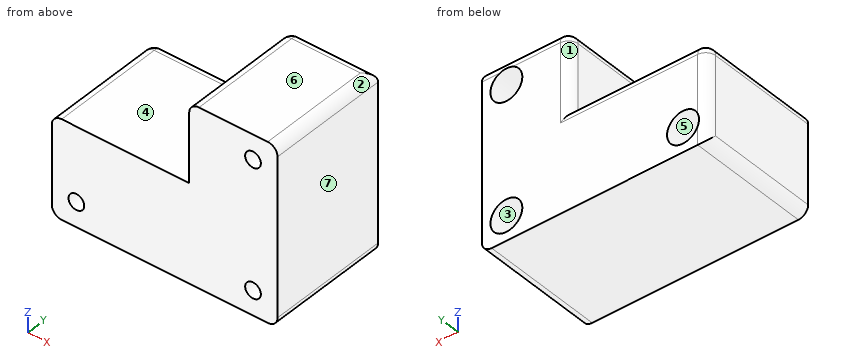
from build123d import *

# Parameters (mm, degrees)
F0_R         = 3.25
F0_R_2       = 1.6
F0_W         = 26
F0_H         = 2
F1_DEPTH     = 25
F2_DEPTH     = 15
F3_T1_DEPTH  = 23
F3_T3_DEPTH  = 21
F3_T5_DEPTH  = 28
F3_T7_DEPTH  = 35
F3_T9_DEPTH  = 26
F3_T11_DEPTH = 14
F3_S15_W     = 2
F3_S15_H     = 2
F3_T16_DEPTH = 2
F3_S21_W     = 2
F3_S21_H     = 2
F3_T22_DEPTH = 2
F3_T29_DEPTH = 31
F3_T33_DEPTH = 19


# Not quite as in the source:
# - a fillet or chamfer that OpenCascade refuses, or shapes differently, is made with other operations: its cross-section is extruded or revolved along the edge and cut away or added


with BuildPart() as f1:
    # F0 (on Front) → F1 (new body)
    with BuildSketch(Plane.XZ):
        Polygon((-23, 0), (-23, -18), (23, -18), (23, 18), (5, 18), (5, 2), (3, 2), (3, 0), align=None)
        with Locations((-18, -13)):
            Circle(F0_R, mode=Mode.SUBTRACT)
        with Locations((18, -13)):
            Circle(F0_R, mode=Mode.SUBTRACT)
        with Locations((18, 13)):
            Circle(F0_R, mode=Mode.SUBTRACT)
        with Locations((18, 13)):
            Circle(F0_R)
        with Locations((18, 13)):
            Circle(F0_R_2, mode=Mode.SUBTRACT)
        with Locations((18, -13)):
            Circle(F0_R)
        with Locations((18, -13)):
            Circle(F0_R_2, mode=Mode.SUBTRACT)
        with Locations((-18, -13)):
            Circle(F0_R)
        with Locations((-18, -13)):
            Circle(F0_R_2, mode=Mode.SUBTRACT)
        with Locations((-10, 1)):
            Rectangle(F0_W, F0_H)
    extrude(amount=F1_DEPTH)

    # F0 (on Front) → F2 (cut)
    with BuildSketch(Plane.XZ):
        with Locations((18, -13)):
            Circle(F0_R)
        with Locations((18, -13)):
            Circle(F0_R_2, mode=Mode.SUBTRACT)
        with Locations((-18, -13)):
            Circle(F0_R)
        with Locations((-18, -13)):
            Circle(F0_R_2, mode=Mode.SUBTRACT)
        with Locations((18, 13)):
            Circle(F0_R)
        with Locations((18, 13)):
            Circle(F0_R_2, mode=Mode.SUBTRACT)
    extrude(amount=F2_DEPTH, mode=Mode.SUBTRACT)

    # F3: fillet of radius 2 on 9 edges, made by hand

    # F3_s2 → F3_t1 (cut)
    with BuildSketch(Plane.XY.offset(-23)):
        with BuildLine():
            ThreePointArc((-23, -2), (-22.4142135624, -0.5857864376), (-21, 0))
            Line((-21, 0), (-23, 0))
            Line((-23, 0), (-23, -2))
        make_face()
    extrude(amount=F3_T1_DEPTH, mode=Mode.SUBTRACT)

    # F3_s4 → F3_t3 (cut)
    with BuildSketch(Plane.YZ.offset(7)):
        with BuildLine():
            ThreePointArc((0, 16), (-0.5857864376, 17.4142135624), (-2, 18))
            Line((-2, 18), (0, 18))
            Line((0, 18), (0, 16))
        make_face()
    extrude(amount=F3_T3_DEPTH, mode=Mode.SUBTRACT)

    # F3_s6 → F3_t5 (cut)
    with BuildSketch(Plane.XZ.offset(2)):
        with BuildLine():
            ThreePointArc((-23, 0), (-22.4142135624, 1.4142135624), (-21, 2))
            Line((-21, 2), (-23, 2))
            Line((-23, 2), (-23, 0))
        make_face()
        with BuildLine():
            ThreePointArc((7, 18), (5.5857864376, 17.4142135624), (5, 16))
            Line((5, 16), (5, 18))
            Line((5, 18), (7, 18))
        make_face()
    extrude(amount=F3_T5_DEPTH, mode=Mode.SUBTRACT)

    # F3_s8 → F3_t7 (cut)
    with BuildSketch(Plane.XZ.offset(-5)):
        with BuildLine():
            ThreePointArc((-21, -18), (-22.4142135624, -17.4142135624), (-23, -16))
            Line((-23, -16), (-23, -18))
            Line((-23, -18), (-21, -18))
        make_face()
        with BuildLine():
            ThreePointArc((21, -18), (22.4142135624, -17.4142135624), (23, -16))
            Line((23, -16), (23, -18))
            Line((23, -18), (21, -18))
        make_face()
        with BuildLine():
            ThreePointArc((23, 16), (22.4142135624, 17.4142135624), (21, 18))
            Line((21, 18), (23, 18))
            Line((23, 18), (23, 16))
        make_face()
    extrude(amount=F3_T7_DEPTH, mode=Mode.SUBTRACT)

    # F3_s10 → F3_t9 (cut)
    with BuildSketch(Plane.YZ.offset(-21)):
        with BuildLine():
            ThreePointArc((0, 0), (-0.5857864376, 1.4142135624), (-2, 2))
            Line((-2, 2), (0, 2))
            Line((0, 2), (0, 0))
        make_face()
    extrude(amount=F3_T9_DEPTH, mode=Mode.SUBTRACT)

    # F3_s12 → F3_t11 (cut)
    with BuildSketch(Plane.XY.offset(2)):
        with BuildLine():
            ThreePointArc((7, 0), (5.5857864376, -0.5857864376), (5, -2))
            Line((5, -2), (5, 0))
            Line((5, 0), (7, 0))
        make_face()
    extrude(amount=F3_T11_DEPTH, mode=Mode.SUBTRACT)


with BuildPart() as f3_tool14:
    # F3_s15 → F3_t16 (new body)
    with BuildSketch(Plane.YZ.offset(-21)):
        with Locations((-1, 1)):
            Rectangle(F3_S15_W, F3_S15_H)
    extrude(amount=-F3_T16_DEPTH)

    # F3_s17 → F3_t18 (revolve, cut)
    with BuildSketch(Plane(origin=(-21, -2, 0), x_dir=(0, -0.7071067812, -0.7071067812), z_dir=(0, 0.7071067812, -0.7071067812))):
        with BuildLine():
            ThreePointArc((0, -2), (2, 0), (0, 2))
            Line((0, 2), (0, -2))
        make_face()
    revolve(axis=Axis((-21, -2, 0), (-1, 0, 0)), mode=Mode.SUBTRACT)


with BuildPart() as f1_1:
    add(f1.part)

    # F3_t13: cut F3_tool14
    add(f3_tool14.part, mode=Mode.SUBTRACT)


with BuildPart() as f3_tool20:
    # F3_s21 → F3_t22 (new body)
    with BuildSketch(Plane.XZ.offset(2)):
        with Locations((6, 17)):
            Rectangle(F3_S21_W, F3_S21_H)
    extrude(amount=-F3_T22_DEPTH)

    # F3_s23 → F3_t24 (revolve, cut)
    with BuildSketch(Plane(origin=(7, -2, 16), x_dir=(0.7071067812, 0, -0.7071067812), z_dir=(0.7071067812, 0, 0.7071067812))):
        with BuildLine():
            ThreePointArc((0, -2), (2, 0), (0, 2))
            Line((0, 2), (0, -2))
        make_face()
    revolve(axis=Axis((7, -2, 16), (0, 1, 0)), mode=Mode.SUBTRACT)


with BuildPart() as f1_2:
    add(f1_1.part)

    # F3_t19: cut F3_tool20
    add(f3_tool20.part, mode=Mode.SUBTRACT)


with BuildPart() as f3_tool27:
    # F3_s28 → F3_t29 (new body)
    with BuildSketch(Plane.YZ.offset(10)):
        with BuildLine():
            ThreePointArc((0, 0), (-0.5857864376, 1.4142135624), (-2, 2))
            Line((-2, 2), (0, 2))
            Line((0, 2), (0, 0))
        make_face()
    extrude(amount=-F3_T29_DEPTH)

    split(bisect_by=Plane.YZ.offset(5), keep=Keep.TOP)


with BuildPart() as f3_tool31:
    # F3_s32 → F3_t33 (new body)
    with BuildSketch(Plane.XY.offset(16)):
        with BuildLine():
            ThreePointArc((7, 0), (5.5857864376, -0.5857864376), (5, -2))
            Line((5, -2), (5, 0))
            Line((5, 0), (7, 0))
        make_face()
    extrude(amount=-F3_T33_DEPTH)

    split(bisect_by=Plane.XY.offset(2), keep=Keep.BOTTOM)


with BuildPart() as f3_tool27_1:
    add(f3_tool27.part)

    # F3_t35: intersect F3_tool31
    add(f3_tool31.part, mode=Mode.INTERSECT)


with BuildPart() as f1_3:
    add(f1_2.part)

    # F3_t25: cut F3_tool27
    add(f3_tool27_1.part, mode=Mode.SUBTRACT)


solid = f1_3.part
The listing builds one solid part. Answer for the finished solid, in the listing's coordinates (mm). Face numbers are marked on the shaded views. A direction names the side the tool comes from. Give positions to 0.01 mm unless a question says otherwise; leave off trailing zeros. Write each loop counter-clockwise with the first axis right and the second up, starting at its lowest first coordinate (ties: lowest second). Pieces come first, ordered by that corner, then holes. Notation, with made-up numbers: (-6, 26) -> (29, 26) arc R24 cw to (29, 43) -> close; hole circle Ø11 at (-22, 27.5). An arc over 180 degrees is marked (long way). Use a Markdown table: item, result.
(1) Flat-ended cylindrical pins translate along their axes: P1, Ø5, axis at x = 6.5, y = -18, coming from the +Z side; P2, Ø2, axis at x = -19, z = -12.5, coming from the +Y side; P3, Ø11.5, axis at x = -1.5, y = -14.5, coming from the +Z side; P4, Ø2.5, axis at x = -18, z = -13, coming from the +Y side. Find the tip coordinate at first contact, or state that the pin passes through.
Return value:
| item | result |
|---|---|
| P1 | z = 18 |
| P2 | y = -15 |
| P3 | z = 2 |
| P4 | through |
(2) Section B-B, the plane y = -5.75 is taken. Determine the outline of the cut face in (x, z).
Return value:
| item | result |
|---|---|
| outline | (-23, -16) arc R2 ccw to (-21, -18) -> (21, -18) arc R2 ccw to (23, -16) -> (23, 16) arc R2 ccw to (21, 18) -> (7, 18) arc R2 ccw to (5, 16) -> (5, 2) -> (-21, 2) arc R2 ccw to (-23, 0) -> close; hole circle Ø6.5 at (-18, -13); hole circle Ø6.5 at (18, -13); hole circle Ø6.5 at (18, 13) |
(3) Section C-C, the plane x = 18 is taken. Determine the outline of the cut face in (y, z).
Return value:
| item | result |
|---|---|
| outline | (-25, -18) -> (0, -18) -> (0, -16.25) -> (-15, -16.25) -> (-15, -14.6) -> (-25, -14.6) -> close; (-25, -11.4) -> (-15, -11.4) -> (-15, -9.75) -> (0, -9.75) -> (0, 9.75) -> (-15, 9.75) -> (-15, 11.4) -> (-25, 11.4) -> close; (-25, 14.6) -> (-15, 14.6) -> (-15, 16.25) -> (-0.02, 16.25) arc R2 ccw to (-2, 18) -> (-25, 18) -> close |
(4) Section D-D, the plane z = -13 is taken. Determine the outline of the cut face in (x, y), then the cut area to 3 significant figures.
Return value:
| item | result |
|---|---|
| outline | (-23, -25) -> (-19.6, -25) -> (-19.6, -15) -> (-21.25, -15) -> (-21.25, -0.02) arc R2 ccw to (-23, -2) -> close; (-16.4, -25) -> (16.4, -25) -> (16.4, -15) -> (14.75, -15) -> (14.75, 0) -> (-14.75, 0) -> (-14.75, -15) -> (-16.4, -15) -> close; (19.6, -25) -> (23, -25) -> (23, 0) -> (21.25, 0) -> (21.25, -15) -> (19.6, -15) -> close |
| area | 890 mm2 |
(5) Find the intervals of material crossed by probe 1 along Z at (x, y) = (18, -22.25); probe 2 along Z at (x, y) = (15, -5.75); probe 3 along X at (y, z) = (-5, 4), in increasing order. Write a range as from..to.
Return value:
| item | result |
|---|---|
| probe 1 | -18..-14.6, -11.4..11.4, 14.6..18 |
| probe 2 | -18..-14.25, -11.75..11.75, 14.25..18 |
| probe 3 | 5..23 |
(6) Determine the mould class of the marked faces 5, 6 and 7 for opening direction X: released by +X, released by -X, zero draft, split by the parting line, or undercut.
Return value:
| item | result |
|---|---|
| face 5 | undercut |
| face 6 | zero draft |
| face 7 | released by +X |
(7) For the marked faces 1, 2, 3 and 4, determine the directions among +Z, -Z, +X, -X, +Y, -Y from which every point of the face is accessible in a straight line to the end or side of a thin tool.
Return value:
| item | result |
|---|---|
| face 1 | +Z, -X, +Y |
| face 2 | +Z, +X, +Y, -Y |
| face 3 | +Y |
| face 4 | +Z, -X, +Y, -Y |
(8) Section A-A, the plane z = 13 is taken. Determine the outline of the cut face in (x, y), then the cut area to 3 significant figures.
Return value:
| item | result |
|---|---|
| outline | (5, -25) -> (16.4, -25) -> (16.4, -15) -> (14.75, -15) -> (14.75, 0) -> (7, 0) arc R2 ccw to (5, -2) -> close; (19.6, -25) -> (23, -25) -> (23, 0) -> (21.25, 0) -> (21.25, -15) -> (19.6, -15) -> close |
| area | 320 mm2 |
